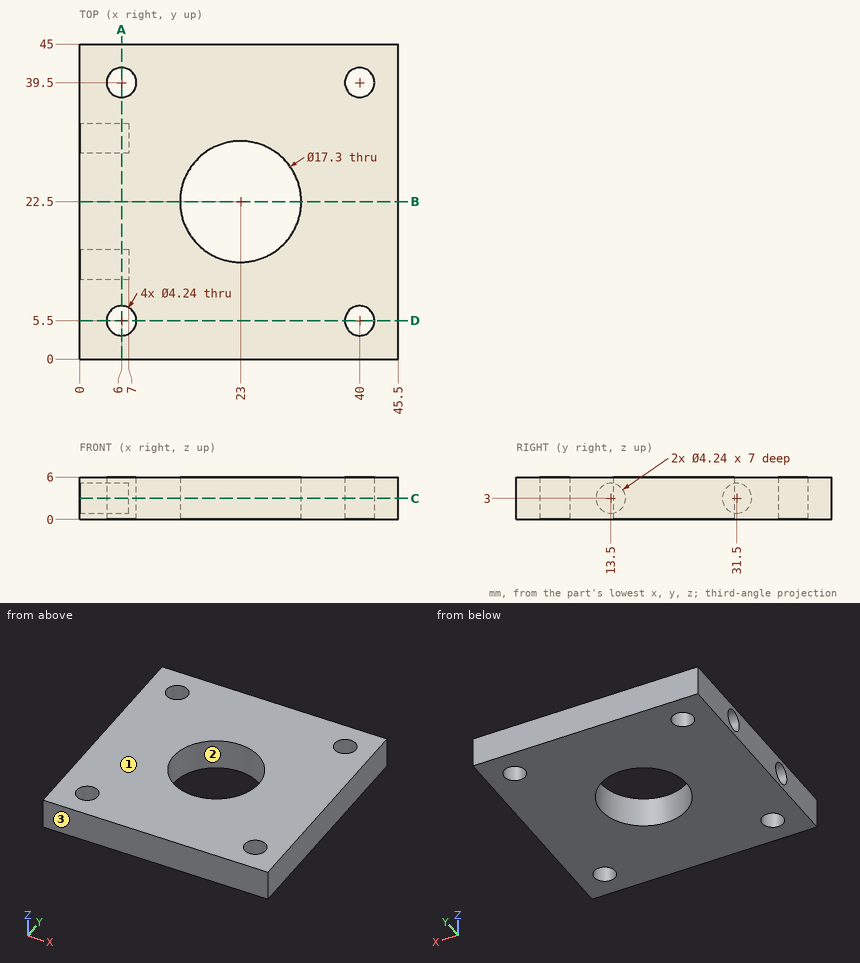
Could you check a few things on this drawing? It's one solid part, dimensions in mm from its lowest x, y, z. Coordinates: 2 decimals unless noted, no trailing zeros. Write each loop counter-clockwise with the first axis right and the second up, starting at its lowest first coordinate (ties: lowest second). Pieces come first, ordered by that corner, then holes.
Q1. If we mould it in two halves opening along Y, with no side actions, what happens to the marked faces 1, 2 and 3? For each: +Y half, -Y half, draft (parallel to the pull), parting line (faces both ways), or undercut.
Results found:
face 1: draft
face 2: undercut
face 3: -Y half
Q2. Please list where these lines run through material, in increasing order: L1, parallel to Y at x = 6, z = 3.1; L2, parallel to Y at x = 40, z = 1.65; L3, parallel to X at y = 38, z = 1.05.
Results found:
L1: y = 0 to 3.38, 7.62 to 11.38, 15.62 to 29.38, 33.62 to 37.38, 41.62 to 45
L2: y = 0 to 3.38, 7.62 to 37.38, 41.62 to 45
L3: x = 0 to 4.5, 7.5 to 38.5, 41.5 to 45.5
Q3. Imagine slicing it at D-D, the plane y = 5.5. List the corners of the cut face in (x, z) for me.
Results found:
outline: (0, 0) - (3.88, 0) - (3.88, 6) - (0, 6) - close; (8.12, 0) - (37.88, 0) - (37.88, 6) - (8.12, 6) - close; (42.12, 0) - (45.5, 0) - (45.5, 6) - (42.12, 6) - close
Q4. For P1, Ø3.5, axis at x = 6, y = 5.5, coming from the +Z side; P2, Ø1.3, axis at y = 12.5, z = 2.5, coming from the -X side, each with a flat end and sliding along its axis, tell me the tip position at first contact or that it passes through.
Results found:
P1: passes through
P2: stops at x = 7
Q5. Imagine slicing it at A-A, the plane x = 6. List the corners of the cut face in (y, z) for me, plus the area to 3 significant figures.
Results found:
outline: (0, 0) - (3.38, 0) - (3.38, 6) - (0, 6) - close; (7.62, 0) - (37.38, 0) - (37.38, 6) - (7.62, 6) - close; (41.62, 0) - (45, 0) - (45, 6) - (41.62, 6) - close; hole circle Ø4.24 at (13.5, 3); hole circle Ø4.24 at (31.5, 3)
area: 191 mm2
Q6. Imagine slicing it at B-B, the plane y = 22.5. List the corners of the cut face in (x, z) for me, plus the area to 3 significant figures.
Results found:
outline: (0, 0) - (14.35, 0) - (14.35, 6) - (0, 6) - close; (31.65, 0) - (45.5, 0) - (45.5, 6) - (31.65, 6) - close
area: 169 mm2
Q7. Imagine slicing it at C-C, the plane z = 3. List the corners of the cut face in (x, y) for me.
Results found:
outline: (0, 0) - (45.5, 0) - (45.5, 45) - (0, 45) - (0, 33.62) - (7, 33.62) - (7, 29.38) - (0, 29.38) - (0, 15.62) - (7, 15.62) - (7, 11.38) - (0, 11.38) - close; hole circle Ø4.24 at (6, 5.5); hole circle Ø4.24 at (6, 39.5); hole circle Ø17.3 at (23, 22.5); hole circle Ø4.24 at (40, 5.5); hole circle Ø4.24 at (40, 39.5)
